```python
from build123d import *

# Parameters (mm, degrees)
F0_R     = 11.43
F0_R_2   = 10.16
F1_DEPTH = 101.6
F3_DEPTH = 12.7


with BuildPart() as f1:
    # F0 (on Top) → F1 (new body)
    with BuildSketch(Plane.XY):
        Circle(F0_R)
        Circle(F0_R_2, mode=Mode.SUBTRACT)
    extrude(amount=F1_DEPTH)


with BuildPart() as f3:
    # F2 (on Right) → F3 (new body, symmetric)
    with BuildSketch(Plane.YZ):
        Polygon((-7.62, 34.2392), (0, 34.2392), (7.62, 34.2392), (7.62, 36.7792), (-7.62, 36.7792), align=None)
    extrude(amount=F3_DEPTH, both=True)


with BuildPart() as f1_1:
    add(f1.part)

    # F4: cut F3
    add(f3.part, mode=Mode.SUBTRACT)


solid = f1_1.part
```
Here's how the part is built. I have some questions about the finished solid (model axes, mm). A direction names the side the tool comes from. Give positions to 0.01 mm unless a question says otherwise; leave off trailing zeros. Write each loop counter-clockwise with the first axis right and the second up, starting at its lowest first coordinate (ties: lowest second). Pieces come first, ordered by that corner, then holes.
(1) On a 3-axis mill with a long thin cutter (end or side, diameter ignored), from which of +Z, -Z, +X, -X, +Y, -Y can I reach the whole of each face in a straight line? I mean faces 1 (the face through (8, 7.62, 35)), 2 (the face through (-8, -7, 0)). Say none if no direction works.
Output values:
face 1: +X, -X
face 2: -Z, +X, -X, +Y, -Y
(2) Thinking about a two-plate mould opening in Z: for faces 3 (the face through (-1.323, 10.074, 50.089)), 4 (the face through (-8, -7, 101.6)), 5 (the face through (8, -7.62, 36)), which applies, pulls with the +Z half, pulls with the -Z half, needs draft (parallel to the pull), parting line crosses it, or undercut?
Output values:
face 3: needs draft
face 4: pulls with the +Z half
face 5: undercut
(3) Imagine slicing it at B-B, the plane y = -6. Write out the boundary of the cut face in (x, z).
Output values:
outline: (-9.73, 0) - (-8.2, 0) - (-8.2, 34.24) - (-9.73, 34.24) - close; (-9.73, 36.78) - (-8.2, 36.78) - (-8.2, 101.6) - (-9.73, 101.6) - close; (8.2, 0) - (9.73, 0) - (9.73, 34.24) - (8.2, 34.24) - close; (8.2, 36.78) - (9.73, 36.78) - (9.73, 101.6) - (8.2, 101.6) - close
(4) Imagine slicing it at A-A, the plane x = 0. Write out the boundary of the cut face in (y, z), and give its area (3 significant figures).
Output values:
outline: (-11.43, 0) - (-10.16, 0) - (-10.16, 101.6) - (-11.43, 101.6) - close; (10.16, 0) - (11.43, 0) - (11.43, 101.6) - (10.16, 101.6) - close
area: 258 mm2
(5) Imagine slicing it at D-D, the plane y = 0. Write out the boundary of the cut face in (x, z).
Output values:
outline: (-11.43, 0) - (-10.16, 0) - (-10.16, 34.24) - (-11.43, 34.24) - close; (-11.43, 36.78) - (-10.16, 36.78) - (-10.16, 101.6) - (-11.43, 101.6) - close; (10.16, 0) - (11.43, 0) - (11.43, 34.24) - (10.16, 34.24) - close; (10.16, 36.78) - (11.43, 36.78) - (11.43, 101.6) - (10.16, 101.6) - close
(6) If I drill on L1, parallel to X at y = 0, z = 75; L2, parallel to Z at x = 10.75, y = 3.5, over which ranges is the centre line in solid material (lowest first)?
Output values:
L1: x = -11.43 to -10.16, 10.16 to 11.43
L2: z = 0 to 34.24, 36.78 to 101.6
(7) Will these pins go through, and if not, where does the flat tip stop? pin 1 (2.5 mm diameter, centred on x = 8, y = -2, fed in from -Z); pin 2 (4 mm diameter, centred on x = -4, z = 78.5, fed in from -Y); pin 3 (3 mm diameter, centred on y = 4, z = 11, fed in from -X); pin 4 (0.5 mm diameter, centred on x = -7.5, z = 35.5, fed in from +Y).
Output values:
pin 1: passes through
pin 2: stops at y = -11.25
pin 3: stops at x = -11.15
pin 4: stops at y = 8.84
(8) Imagine slicing it at C-C, the plane z = 21. Write out the boundary of the cut face in (x, y).
Output values:
outline: circle Ø22.86 at (0, 0); hole circle Ø20.32 at (0, 0)
